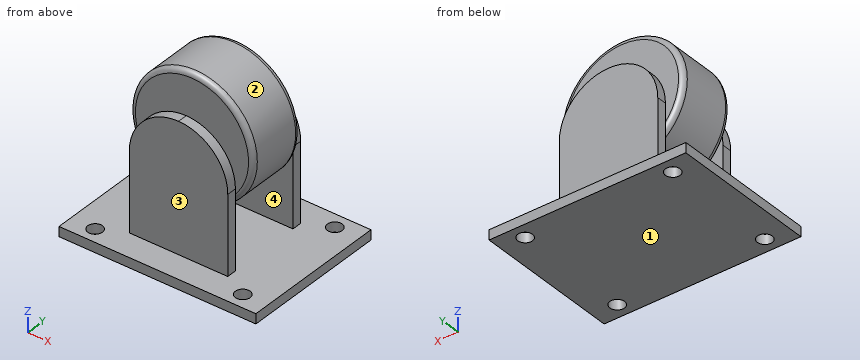
from build123d import *

# Parameters (mm, degrees)
SKETCH1_W                = 40
SKETCH1_H                = 30
BOSS_EXTRUDE1_DEPTH      = 2
SKETCH2_R                = 1.5
CUT_EXTRUDE1_DEPTH       = 26.079872408
SKETCH3_W                = 20
SKETCH3_H                = 2
BOSS_EXTRUDE2_DEPTH      = 26
SKETCH4_R                = 2.5
BOSS_EXTRUDE3_DEPTH      = 19
BOSS_EXTRUDE4_DEPTH      = 6
BOSS_EXTRUDE4_DEPTH_BACK = 6
SKETCH5_R                = 12.5
FILLET1_R                = 10
FILLET2_R                = 1


with BuildPart() as part:
    # Sketch1 → Boss-Extrude1 (new body)
    with BuildSketch(Plane.XY):
        Rectangle(SKETCH1_W, SKETCH1_H)
    extrude(amount=BOSS_EXTRUDE1_DEPTH)

    # Sketch2 → Cut-Extrude1 (cut, through all)
    with BuildSketch(Plane.XY.offset(2)):
        with Locations((-15, 12)):
            Circle(SKETCH2_R)
        with Locations((15, 12)):
            Circle(SKETCH2_R)
        with Locations((15, -12)):
            Circle(SKETCH2_R)
        with Locations((-15, -12)):
            Circle(SKETCH2_R)
    extrude(amount=-CUT_EXTRUDE1_DEPTH, mode=Mode.SUBTRACT)

    # Sketch3 → Boss-Extrude2 (add)
    with BuildSketch(Plane.XY.offset(2)):
        with Locations((0, -8.5)):
            Rectangle(SKETCH3_W, SKETCH3_H)
        with Locations((0, 8.5)):
            Rectangle(SKETCH3_W, SKETCH3_H)
    extrude(amount=BOSS_EXTRUDE2_DEPTH)

    # Sketch4 → Boss-Extrude3 (add)
    with BuildSketch(Plane(origin=(0, 9.5, 0), x_dir=(1, 0, 0), z_dir=(0, 1, 0))):
        with Locations(Location((0, -23, 0), (0, 0, 270))):
            Circle(SKETCH4_R)
    extrude(amount=-BOSS_EXTRUDE3_DEPTH)

    # Sketch5 → Boss-Extrude4 (add, two sides: drawn at the far end of the back side and taken through both)
    with BuildSketch(Plane(origin=(0, 0, 0), x_dir=(-1, 0, 0), z_dir=(0, -1, 0)).offset(-BOSS_EXTRUDE4_DEPTH_BACK)):
        with Locations(Location((0, -23, 0), (0, 0, 90))):
            Circle(SKETCH5_R)
    extrude(amount=BOSS_EXTRUDE4_DEPTH + BOSS_EXTRUDE4_DEPTH_BACK)

    # Fillet1
    fillet1_edges = [part.edges().sort_by_distance(p)[0] for p in [
        (10, -8.5, 28),
        (-10, -8.5, 28),
        (10, 8.5, 28),
        (-10, 8.5, 28),
    ]]
    fillet(fillet1_edges, radius=FILLET1_R - 0.0001)  # a hair under: the kernel refuses the full size

    # Fillet2
    fillet2_edges = [part.edges().sort_by_distance(p)[0] for p in [
        (0, 6, 35.5),
        (0, -6, 35.5),
    ]]
    fillet(fillet2_edges, radius=FILLET2_R)


solid = part.part
Verification items for the finished model (mm, model axes). Face numbers are marked on the shaded views. Coordinates: 2 decimals unless noted, no trailing zeros. Order: outer loops, then holes, each group sorted by start corner. A loop starts at its lowest first (then second) coordinate and runs counter-clockwise, first axis right, second up.
Item 1: Section check D-D, the plane z = 3. Enter the section's corners in (x, y), then the cut area to 3 significant figures.
Filled in:
outline: (-10, -9.5) - (10, -9.5) - (10, -7.5) - (-10, -7.5) - close; (-10, 7.5) - (10, 7.5) - (10, 9.5) - (-10, 9.5) - close
area: 80.0 mm2
Item 2: Section check C-C, the plane y = 2.75. Enter the section's corners in (x, z).
Filled in:
outline: (-20, 0) - (20, 0) - (20, 2) - (-20, 2) - close; circle Ø25 at (0, 23)
Item 3: Material ranges on L1, parallel to Y at x = 6.5, z = 16.5; L2, parallel to Y at x = -15, z = 0.5; L3, parallel to Y at x = 2, z = 7.5, recorded low to high.
Filled in:
L1: y = -9.5 to -7.5, -6 to 6, 7.5 to 9.5
L2: y = -15 to -13.5, -10.5 to 10.5, 13.5 to 15
L3: y = -9.5 to -7.5, 7.5 to 9.5
Item 4: Section check B-B, the plane x = 15. Enter the section's corners in (y, z).
Filled in:
outline: (-15, 0) - (-13.5, 0) - (-13.5, 2) - (-15, 2) - close; (-10.5, 0) - (10.5, 0) - (10.5, 2) - (-10.5, 2) - close; (13.5, 0) - (15, 0) - (15, 2) - (13.5, 2) - close
Item 5: Release check for a two-part mould opening along Z. For the marked faces 1, 2, 3 and 4 record: +Z half, -Z half, draft (parallel to the pull), parting line (faces both ways), or undercut.
Filled in:
face 1: -Z half
face 2: undercut
face 3: draft
face 4: undercut
Item 6: Section check A-A, the plane y = -12. Enter the section's corners in (x, z).
Filled in:
outline: (-20, 0) - (-16.5, 0) - (-16.5, 2) - (-20, 2) - close; (-13.5, 0) - (13.5, 0) - (13.5, 2) - (-13.5, 2) - close; (16.5, 0) - (20, 0) - (20, 2) - (16.5, 2) - close
Item 7: Depth check by flat-ended pin: pin 1 (1 mm diameter, centred on y = -9, z = 7.5, fed in from +X); pin 2 (1.5 mm diameter, centred on x = -11, y = -10, fed in from +Z); pin 3 (12 mm diameter, centred on x = -4.5, z = 9.5, fed in from +Y); pin 4 (2.5 mm diameter, centred on x = -15, y = -12, fed in from -Z). Enter the tip coordinate at first touch or a pass-through.
Filled in:
pin 1: stops at x = 10
pin 2: stops at z = 2
pin 3: stops at y = 9.5
pin 4: passes through
